from build123d import *

# Parameters (mm, degrees)
SKETCH1_R           = 63.5
BOSS_EXTRUDE1_DEPTH = 812.8
SKETCH2_R           = 71.128555951
BOSS_EXTRUDE2_DEPTH = 12.7


with BuildPart() as part:
    # Sketch1 → Boss-Extrude1 (new body)
    with BuildSketch(Plane(origin=(0, 0, 0), x_dir=(1, 0, 0), z_dir=(0, 1, 0))):
        with Locations(Location((0, 0, 0), (0, 0, 270))):
            Circle(SKETCH1_R)
    extrude(amount=BOSS_EXTRUDE1_DEPTH)

    # Sketch2 → Boss-Extrude2 (add)
    with BuildSketch(Plane(origin=(0, 812.8, 0), x_dir=(1, 0, 0), z_dir=(0, 1, 0))):
        with Locations(Location((0, 0, 0), (0, 0, 270))):
            Circle(SKETCH2_R)
    extrude(amount=BOSS_EXTRUDE2_DEPTH)

    # Sketch5 → Revolve2 (revolve)
    with BuildSketch(Plane(origin=(0, 0, 0), x_dir=(0, 0, -1), z_dir=(1, 0, 0))):
        Polygon((-63.5, 0), (0, 0), (0, -223.940998137), (-4.689426477, -223.940998137), align=None)
    revolve(axis=Axis((0, 0, 0), (0, -1, 0)))


solid = part.part
Geometry: final body of the model. Coordinates: model frame, mm. Coordinates: 2 decimals unless noted, no trailing zeros. Loops run counter-clockwise (first coordinate to the right, second up) from the corner with the lowest first, then second, coordinate; pieces in that order, holes last. Notation, with made-up numbers: M 56.5,13 L 61.5,13 A27 ccw 61.5,31 Z; hole C -6,-16 d4. An arc over 180 degrees is marked long. One line per item, written item: value. Start each with the question number.
1) Cut plane A-A (y = 397). Return loops of the section in (x, z).
2) Cut plane B-B (y = -136.5). Return loops of the section in (x, z).
3) Material intervals for L1, parallel to Z at x = -2.5, y = 283; L2, parallel to Y at x = 33.5, z = -57; L3, parallel to X at y = 325, z = 7.5, sorted ascending. Write a range as from..to.
4) Draft query along Y for faces 1 (the flat face through (1, 825.5, -1)), 2 (the flat face through (58, 812.8, -27)), 3 (the cylindrical face through (-61.99, 400.71, -13.77)). Return one class per face: released by +Y, released by -Y, zero draft, split by the parting line, or undercut.
5) Pin query (flat end, axial travel): P1, Ø12, axis at x = -48, y = 520, coming from the -Z side; P2, Ø12, axis at y = 29.5, z = -22, coming from the -X side; P3, Ø6, axis at x = -37.5, y = 647.5, coming from the +Z side. Return the tip coordinate at first contact, or that it passes through.
Evaluation:
1. outline: C 0,0 d127
2. outline: C 0,0 d55.31
3. L1: -63.45..63.45
3. L2: 812.8..825.5
3. L3: -63.06..63.06
4. face 1: released by +Y
4. face 2: released by -Y
4. face 3: zero draft
5. P1: z = -47.63
5. P2: x = -61.45
5. P3: z = 53.31
